from build123d import *
from build123d.topology import SkipClean

# Parameters (mm, degrees)
SALIENTE_EXTRUIR1_DEPTH = 3.5
CROQUIS2_R              = 1.5
CORTAR_EXTRUIR1_DEPTH   = 7
CROQUIS3_R              = 4
CROQUIS3_R_2            = 3
SALIENTE_EXTRUIR2_DEPTH = 5


with BuildPart() as part:
    # Croquis1 → Saliente-Extruir1 (new, symmetric)
    with SkipClean():  # the faces are left unmerged after this step: merging them gives an invalid solid
        with BuildSketch(Plane(origin=(0, 0, 0), x_dir=(1, 0, 0), z_dir=(0, 1, 0))):
            with BuildLine():
                Line((35, 0), (18, 0))
                ThreePointArc((18, 0), (0, -18), (-18, 0))
                Line((-18, 0), (-50, 0))
                ThreePointArc((-50, 0), (-17.044661679, -47.005100875), (38.37918033, -32.047441664))
                ThreePointArc((38.37918033, -32.047441664), (38.439227262, -31.49182987), (37.949409202, -31.222779006))
                ThreePointArc((37.949409202, -31.222779006), (35.879823326, -30.517678888), (35, -28.516113802))
                Line((35, -28.516113802), (35, 0))
            make_face()
            with BuildLine():
                ThreePointArc((-18, 0), (0, 18), (18, 0))
                Line((18, 0), (35, 0))
                Line((35, 0), (35, 28.516113802))
                ThreePointArc((35, 28.516113802), (35.879823326, 30.517678888), (37.949409202, 31.222779006))
                ThreePointArc((37.949409202, 31.222779006), (38.439227262, 31.49182987), (38.37918033, 32.047441664))
                ThreePointArc((38.37918033, 32.047441664), (36.735192641, 33.919398898), (35, 35.707142143))
                ThreePointArc((35, 35.707142143), (-19.364916731, 46.097722286), (-50, 0))
                Line((-50, 0), (-18, 0))
            make_face()
        extrude(amount=SALIENTE_EXTRUIR1_DEPTH, both=True)

    # Croquis2 → Cortar-Extruir1 (cut)
    with SkipClean():  # the faces are left unmerged after this step: merging them gives an invalid solid
        with BuildSketch(Plane.XZ.offset(3.5)):
            with Locations(Location((17.5, 30.310889132, 0), (0, 0, 270))):
                Circle(CROQUIS2_R)
            with Locations(Location((-35, 0, 0), (0, 0, 270))):
                Circle(CROQUIS2_R)
            with Locations(Location((17.5, -30.310889132, 0), (0, 0, 270))):
                Circle(CROQUIS2_R)
        extrude(amount=-CORTAR_EXTRUIR1_DEPTH, mode=Mode.SUBTRACT)

    # Croquis3 → Saliente-Extruir2 (add)
    # profile 1 of 3: a face of its own
    with SkipClean():  # the faces are left unmerged after this step: merging them gives an invalid solid
        with BuildSketch(Plane.XZ.offset(3.5)):
            with Locations(Location((-35, 0, 0), (0, 0, 90))):
                Circle(CROQUIS3_R)
            with Locations(Location((-35, 0, 0), (0, 0, 270))):
                Circle(CROQUIS3_R_2, mode=Mode.SUBTRACT)
        # profile 2 of 3: a face of its own
        with BuildSketch(Plane.XZ.offset(3.5)):
            with Locations(Location((17.5, 30.310889132, 0), (0, 0, 90))):
                Circle(CROQUIS3_R)
            with Locations(Location((17.5, 30.310889132, 0), (0, 0, 270))):
                Circle(CROQUIS3_R_2, mode=Mode.SUBTRACT)
        # profile 3 of 3: a face of its own
        with BuildSketch(Plane.XZ.offset(3.5)):
            with Locations(Location((17.5, -30.310889132, 0), (0, 0, 90))):
                Circle(CROQUIS3_R)
            with Locations(Location((17.5, -30.310889132, 0), (0, 0, 270))):
                Circle(CROQUIS3_R_2, mode=Mode.SUBTRACT)
        extrude(amount=SALIENTE_EXTRUIR2_DEPTH)


solid = part.part
Geometry check sheet. Reference: the model listing, model coordinates, mm. A direction names the side the tool comes from. Give positions to 0.01 mm unless a question says otherwise; leave off trailing zeros. Write each loop counter-clockwise with the first axis right and the second up, starting at its lowest first coordinate (ties: lowest second). Pieces come first, ordered by that corner, then holes. Notation, with made-up numbers: (-36.5, -18.5) - (12.5, -18.5) arc R20 ccw to (12.5, -3.5) - close; hole circle Ø4 at (-32, 82.25). An arc over 180 degrees is marked (long way). Put each result on its own line as item: value.
1. Sectioned sample at D-D, the plane x = -35. Enter the section's corners in (y, z), plus the area to 3 significant figures.
Ans:
outline: (-8.5, -4) - (-3.5, -4) - (-3.5, -35.71) - (3.5, -35.71) - (3.5, -1.5) - (-3.5, -1.5) - (-3.5, -3) - (-8.5, -3) - close; (-8.5, 3) - (-3.5, 3) - (-3.5, 1.5) - (3.5, 1.5) - (3.5, 35.71) - (-3.5, 35.71) - (-3.5, 4) - (-8.5, 4) - close
area: 489 mm²
2. Sectioned sample at C-C, the plane z = 6. Enter the section's corners in (x, y).
Ans:
outline: (-49.64, -3.5) - (-16.97, -3.5) - (-16.97, 3.5) - (-49.64, 3.5) - close; (16.97, -3.5) - (35, -3.5) - (35, 3.5) - (16.97, 3.5) - close
3. Sectioned sample at A-A, the plane y = -5. Enter the section's corners in (x, z), plus the area to 3 significant figures.
Ans:
outline: circle Ø8 at (-35, 0); circle Ø8 at (17.5, -30.31); circle Ø8 at (17.5, 30.31); hole circle Ø6 at (-35, 0); hole circle Ø6 at (17.5, -30.31); hole circle Ø6 at (17.5, 30.31)
area: 66.0 mm²
4. Draft check along X on faces 3 (the cylindrical face through (15.675, -5.965, -27.93)), 4 (the cylindrical face through (-38.966, -5.965, -0.521)), 5 (the flat face through (18, -8.5, 27)). Enter one of: +X half, -X half, draft (parallel to the pull), parting line (faces both ways), or undercut.
Ans:
face 3: undercut
face 4: parting line
face 5: draft
5. Go/stop test with flat-tipped pins: pin 1 (2.5 mm diameter, centred on x = -35, z = 0, fed in from -Y); pin 2 (8 mm diameter, centred on x = -7.5, z = -36.5, fed in from -Y); pin 3 (3.5 mm diameter, centred on x = 17.5, z = 30.31, fed in from +Y); pin 4 (4 mm diameter, centred on y = 1, z = 20.5, fed in from +X). Record where each tip stops, or that it passes through.
Ans:
pin 1: passes through
pin 2: stops at y = -3.5
pin 3: stops at y = 3.5
pin 4: stops at x = 35
6. Thickness scan on line 1 (Z direction, x = -35, y = -6.35); line 2 (Z direction, x = 20, y = -6.25); line 3 (Y direction, x = -27.5, z = -27.5). Record the ranges inside material, lowest first.
Ans:
line 1: z = -4 to -3, 3 to 4
line 2: z = -33.43 to -31.97, -28.65 to -27.19, 27.19 to 28.65, 31.97 to 33.43
line 3: y = -3.5 to 3.5
7. Set-up check for faces 1 (the cylindrical face through (18.76, -0.05, 29.5)), 2 (the cylindrical face through (17.63, -5.96, 33.31)): record each of +Z, -Z, +X, -X, +Y, -Y from which the full face is reachable in a straight line by a thin tool's end or side.
Ans:
face 1: +Y, -Y
face 2: -Y
8. Sectioned sample at B-B, the plane x = 0. Enter the section's corners in (y, z).
Ans:
outline: (-3.5, -50) - (3.5, -50) - (3.5, -18) - (-3.5, -18) - close; (-3.5, 18) - (3.5, 18) - (3.5, 50) - (-3.5, 50) - close
